from build123d import *

# Parameters (mm, degrees)
SKETCH1_W           = 12
SKETCH1_H           = 23
BOSS_EXTRUDE1_DEPTH = 22
CHAMFER1_SIZE       = 4
CHAMFER1_SIZE2      = 6.92820323
BOSS_EXTRUDE2_DEPTH = 2
SKETCH3_R           = 6
BOSS_EXTRUDE3_DEPTH = 4
SKETCH4_W           = 5.5
SKETCH4_H           = 8.3
BOSS_EXTRUDE4_DEPTH = 3
SKETCH5_R           = 1.15
BOSS_EXTRUDE5_DEPTH = 1
SKETCH6_R           = 2.375
SKETCH6_R_2         = 0.5
BOSS_EXTRUDE6_DEPTH = 3.5
CHAMFER2_SIZE       = 1
CHAMFER2_SIZE2      = 7.115369722


with BuildPart() as part:
    # Sketch1 → Boss-Extrude1 (new body)
    with BuildSketch(Plane(origin=(0, 0, 0), x_dir=(1, 0, 0), z_dir=(0, 1, 0))):
        with Locations((0, -5.5)):
            Rectangle(SKETCH1_W, SKETCH1_H)
    extrude(amount=BOSS_EXTRUDE1_DEPTH)

    # Chamfer1
    chamfer1_edges = [part.edges().sort_by_distance(p)[0] for p in [
        (0, 0, -6),
    ]]
    chamfer1_side = [part.faces().sort_by_distance(p)[0] for p in [
        (0, 11, -6),
    ]]
    chamfer(chamfer1_edges, length=CHAMFER1_SIZE, length2=CHAMFER1_SIZE2, reference=chamfer1_side[0])

    # Sketch2 → Boss-Extrude2 (add)
    with BuildSketch(Plane(origin=(0, 16, 0), x_dir=(-1, 0, 0), z_dir=(0, 1, 0))):
        with BuildLine():
            Line((6, -6), (6, -10.5))
            Line((6, -10.5), (1.54029218, -10.5))
            ThreePointArc((1.54029218, -10.5), (0, -6.85), (-1.54029218, -10.5))
            Line((-1.54029218, -10.5), (-6, -10.5))
            Line((-6, -10.5), (-6, -6))
            Line((-6, -6), (6, -6))
        make_face()
        with BuildLine():
            Line((-6, 21.5), (-1.54029218, 21.5))
            ThreePointArc((-1.54029218, 21.5), (0, 17.85), (1.54029218, 21.5))
            Line((1.54029218, 21.5), (6, 21.5))
            Line((6, 21.5), (6, 17))
            Line((6, 17), (-6, 17))
            Line((-6, 17), (-6, 21.5))
        make_face()
    extrude(amount=BOSS_EXTRUDE2_DEPTH)

    # Sketch3 → Boss-Extrude3 (add)
    with BuildSketch(Plane(origin=(0, 22, 0), x_dir=(1, 0, 0), z_dir=(0, 1, 0))):
        Circle(SKETCH3_R)
    extrude(amount=BOSS_EXTRUDE3_DEPTH)

    # Sketch4 → Boss-Extrude4 (add)
    with BuildSketch(Plane(origin=(0, 22, 0), x_dir=(1, 0, 0), z_dir=(0, 1, 0))):
        with Locations((0, -4.15)):
            Rectangle(SKETCH4_W, SKETCH4_H)
    extrude(amount=BOSS_EXTRUDE4_DEPTH)

    # Sketch5 → Boss-Extrude5 (add)
    with BuildSketch(Plane(origin=(0, 25, 0), x_dir=(1, 0, 0), z_dir=(0, 1, 0))):
        with Locations((0, -6)):
            Circle(SKETCH5_R)
    extrude(amount=BOSS_EXTRUDE5_DEPTH)

    # Sketch6 → Boss-Extrude6 (add)
    with BuildSketch(Plane(origin=(0, 26, 0), x_dir=(1, 0, 0), z_dir=(0, 1, 0))):
        Circle(SKETCH6_R)
        Circle(SKETCH6_R_2, mode=Mode.SUBTRACT)
    extrude(amount=BOSS_EXTRUDE6_DEPTH)

    # Chamfer2
    chamfer2_edges = [part.edges().sort_by_distance(p)[0] for p in [
        (0, 22, 17),
    ]]
    chamfer2_side = [part.faces().sort_by_distance(p)[0] for p in [
        (0, 20, 17),
    ]]
    chamfer(chamfer2_edges, length=CHAMFER2_SIZE, length2=CHAMFER2_SIZE2, reference=chamfer2_side[0])


solid = part.part
Verification items for the finished model (mm, model axes). A direction names the side the tool comes from. Coordinates: 2 decimals unless noted, no trailing zeros. Order: outer loops, then holes, each group sorted by start corner. A loop starts at its lowest first (then second) coordinate and runs counter-clockwise, first axis right, second up. Notation, with made-up numbers: M 27,48 L 72,48 A20 cw 72,56 Z; hole C -27.5,83.5 d1. An arc over 180 degrees is marked long. One line per item, written item: value. Start each with the question number.
Item 1: Sectioned sample at C-C on y = 20.5. Record the cut outline in (x, z), then the cut area to 3 significant figures.
Item 2: Sectioned sample at D-D on z = 9. Record the cut outline in (x, y), then the cut area to 3 significant figures.
Item 3: Depth check by flat-ended pin: P1, Ø3, axis at x = 4, y = 11, coming from the -Z side; P2, Ø2, axis at x = 3, y = 9.5, coming from the +Z side; P3, Ø5, axis at x = 0, z = -9, coming from the -Y side; P4, Ø4, axis at x = 0, z = 20, coming from the +Y side. Enter the tip coordinate at first touch or a pass-through.
Item 4: Thickness scan on probe 1 along Z at (x, y) = (0, 28.2) (3 decimals); probe 2 along X at (y, z) = (16.75, 20). Record the ranges inside material, lowest first.
Item 5: Access from +Z, -Z, +X, -X, +Y, -Y to the whole of each face (thin tool, end or side, straight path). Record for faces 1 (the flat face through (-0.1, 18, 17.3)), 2 (the flat face through (-0.1, 16, -6.7)), 3 (the flat face through (-0.1, 16, 17.3)), 4 (the cylindrical face through (0, 24, -6)).
Item 6: Sectioned sample at B-B on x = 4.5. Record the cut outline in (y, z), then the cut area to 3 significant figures.
Item 7: Sectioned sample at A-A on z = 20. Record the cut outline in (x, y), then the cut area to 3 significant figures.
Calculated:
1. outline: M -6,-6 L 6,-6 L 6,17 L -6,17 Z
1. area: 276 mm^2
2. outline: M -6,0 L 6,0 L 6,22 L -6,22 Z
2. area: 264 mm^2
3. P1: z = -6
3. P2: z = 17
3. P3: y = 16
3. P4: through
4. probe 1: -2.375 to -0.5, 0.5 to 2.375
4. probe 2: -6 to -2.15, 2.15 to 6
5. face 1: +Z, +X, -X, +Y
5. face 2: -Z, +X, -X, -Y
5. face 3: +Z, +X, -X, -Y
5. face 4: +Y
6. outline: M 0,0.93 L 4,-6 L 16,-6 L 16,-10.5 L 18,-10.5 L 18,-6 L 22,-6 L 22,-3.97 L 26,-3.97 L 26,3.97 L 22,3.97 L 22,9.88 L 21,17 L 18,17 L 18,21.5 L 16,21.5 L 16,17 L 0,17 Z
6. area: 538 mm^2
7. outline: M -6,16 L -2.15,16 L -2.15,18 L -6,18 Z; M 2.15,16 L 6,16 L 6,18 L 2.15,18 Z
7. area: 15.4 mm^2
